Could you check a few things on this model? Use its own coordinates, in mm. Face numbers are marked on the shaded views. A direction names the side the tool comes from. Give positions to 0.01 mm unless a question says otherwise; leave off trailing zeros. Order: outer loops, then holes, each group sorted by start corner. A loop starts at its lowest first (then second) coordinate and runs counter-clockwise, first axis right, second up. Notation, with made-up numbers: M 38.25,84.5 L 53.25,84.5 A29 cw 53.25,110.5 Z; hole C 89.5,-18 d9. An arc over 180 degrees is marked long. Use a Markdown table: item, result. Add a question column.
Item 1: Suppose I cut it at A-A on z = -4. Write out the boundary of the cut face in (x, y), plus the area to 3 significant figures.
Item 2: Suppose I cut it at D-D on y = -12.5. Write out the boundary of the cut face in (x, z), plus the area to 3 significant figures.
Item 3: For the marked faces 1, 2 and 3, which set-ups out of +Z, -Z, +X, -X, +Y, -Y let a thin tool reach every point of the face, with its end or its side?
Item 4: Suppose I cut it at C-C on x = -9.5. Write out the boundary of the cut face in (y, z).
Item 5: If I drill on L1, parallel to Y at x = -12.9, z = -4; L2, parallel to Y at x = -1.25, z = 3; L3, parallel to X at y = -18.5, z = 0, over which ranges is the centre line in solid material (lowest first)? Write a range as from..to.
Item 6: Suppose I cut it at B-B on z = -7. Write out the boundary of the cut face in (x, y).
Item 7: I'm going to push flat-ended pins straight in: pin 1 Ø3 at (x, y) = (-6.31, 1.14) entering from -Z; pin 2 Ø2 at (x, y) = (-13.5, -30) entering from +Z; pin 3 Ø2 at (x, z) = (-9, 2) entering from -Y. Where does each tip first touch, or does it pass through?
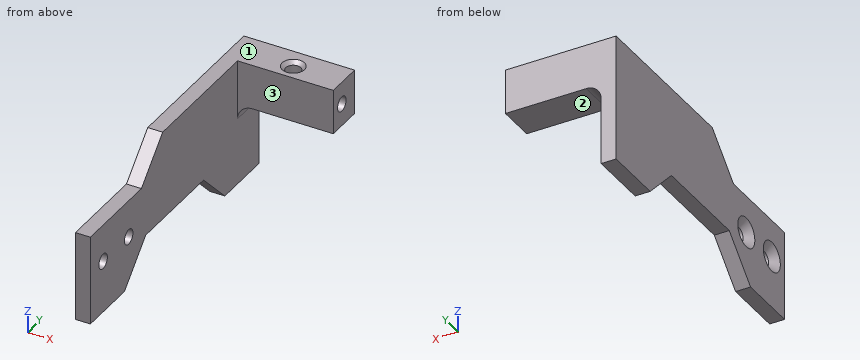
Autodesk Inventor part; units mm, degrees
ref_plane "YZ Plane" through (0, 0, 0) normal (1, 0, 0) x (0, 1, 0)
ref_plane "XZ Plane" through (0, 0, 0) normal (0, 1, 0) x (-1, 0, 0)
ref_plane "XY Plane" through (0, 0, 0) normal (0, 0, 1) x (1, 0, 0)
sketch "Sketch1" plane through (0, 0, 0) normal (0, 0, 1) x (1, 0, 0)
  line L0 (-12.5097, 3.9382) -> (-0.5097, 3.9382)
  line L1 (-0.5097, 3.9382) -> (-0.5097, -1.0618)
  line L2 (-0.5097, -1.0618) -> (-12.5097, -1.0618)
  line L3 (-12.5097, -1.0618) -> (-12.5097, 3.9382)
  point P0 (0, 0)
  dimension "d0" = 12
  dimension "d1" = 5
extrude "Extrusion1" add sketch "Sketch1" along normal blind 6
sketch "Sketch2" plane through (0, 0, 6) normal (0, 0, 1) x (1, 0, 0)
  line L0 (-0.5097, -1.0618) -> (-0.5097, 3.9382)
  line L1 (-0.5097, 3.9382) -> (-12.5097, 3.9382)
  point P0 (0, 0)
  point P1 (-6.3097, 1.1382)
  dimension "d4" = 5.8
  dimension "d5" = 2.8
hole "Hole1" at (-6.3097, 1.1382, 6) direction (0, 0, -1) diameter 2 depth 5 tip angle 118 countersink diameter 3 countersink angle 90
sketch "Sketch3" plane through (-0.5097, -1.0618, 0) normal (1, 0, 0) x (0, 0, -1)
  line L0 (0, 5) -> (-6, 5)
  line L1 (-6, 0) -> (-6, 5)
  point P0 (0, 1.0618)
  point P1 (-3, 2)
  dimension "d13" = 3
  dimension "d14" = 3
hole "Hole2" at (-0.5097, 0.9382, 3) direction (-1, 0, 0) diameter 2 depth 3 tip angle 118
sketch "Sketch4" plane through (-12.5097, -1.0618, 0) normal (-1, 0, 0) x (0, 0, 1)
  line L0 (6, 0) -> (6, 5)
  line L1 (6, 5) -> (-11, 5)
  line L2 (-11, 5) -> (-11, -34.6)
  line L3 (-11, -34.6) -> (6, -34.6)
  line L4 (6, -34.6) -> (6, 5)
  point P0 (0, 1.0618)
  dimension "d22" = 17
  dimension "d23" = 39.6
extrude "Extrusion2" add sketch "Sketch4" along normal blind 2
sketch "Sketch5" plane through (-14.5097, -1.0618, 0) normal (-1, 0, 0) x (0, 0, 1)
  line L0 (-11, -34.6) -> (6, -34.6)
  line L1 (6, -34.6) -> (6, 5)
  point P0 (0, 1.0618)
  point P1 (-4, -25.6)
  point P2 (-4, -31.6)
  dimension "d26" = 3
  dimension "d27" = 9
  dimension "d28" = 10
  dimension "d29" = 10
hole "Hole3" at (-14.5097, -26.6618, -4) at (-14.5097, -32.6618, -4) direction (1, 0, 0) diameter 2 depth 3 tip angle 118 countersink diameter 4 countersink angle 90
sketch "Sketch6" plane through (-0.5097, -1.0618, 0) normal (1, 0, 0) x (0, 0, -1)
  line L0 (-6, 5) -> (11, 5)
  line L1 (0, 5) -> (0, 0)
  line L2 (-6, 5) -> (0, 5)
  line L3 (0, 5) -> (0, 0)
  line L4 (0, 0) -> (-6, 0)
  line L5 (-6, 0) -> (-6, 5)
  circle A0 centre (-3, 2) radius 1
  circle A1 centre (-3, 2) radius 1
  point P0 (0, 1.0618)
  dimension "d37" = 2
extrude "Extrusion3" add sketch "Sketch6" along normal blind 0.8
sketch "Sketch7" plane through (-14.5097, -35.6618, 6) normal (-1, 0, 0) x (0, 0, 1)
  line L0 (-17, 39.6) -> (-17, 0)
  line L1 (-17, 31.6) -> (-12, 31.6)
  line L2 (-12, 31.6) -> (-12, 8)
  line L3 (-12, 8) -> (-17, 8)
  line L4 (-17, 8) -> (-17, 31.6)
  line L5 (0, 39.6) -> (-17, 39.6)
  line L6 (-17, 0) -> (0, 0)
  point P0 (-6, 35.6618)
  point P1 (-10, 0)
  point P2 (-17, 8)
  dimension "d40" = 5
  dimension "d41" = 8
  dimension "d42" = 8
extrude "Extrusion4" cut sketch "Sketch7" against normal blind 2
chamfer "Chamfer1" distance 5 angle 45 2 edges at (-13.5097, -4.0618, -6) (-13.5097, -27.6618, -6)
fillet "Fillet1" radius 2 1 edges at (-12.5097, 1.4382, 0)
sketch "Sketch8" plane through (-14.5097, -35.6618, 6) normal (-1, 0, 0) x (0, 0, 1)
  line L0 (0, 0) -> (0, 39.6)
  line L1 (-17, 0) -> (0, 0)
  line L2 (0, 12) -> (-5, 12)
  line L3 (-5, 12) -> (-5, 0)
  line L4 (-5, 0) -> (0, 0)
  line L5 (0, 0) -> (0, 12)
  point P0 (-6, 35.6618)
  point P1 (-10, 0)
  dimension "d49" = 5
  dimension "d50" = 12
extrude "Extrusion5" cut sketch "Sketch8" against normal blind 10
chamfer "Chamfer2" distance 5 angle 45 1 edges at (-13.5097, -23.6618, 6)
properties part number "servo-mount"
Findings below:
| question | item | result |
|---|---|---|
| 1 | outline | M -14.51,-35.66 L -12.51,-35.66 L -12.51,-33.66 L -13.51,-33.66 L -14.51,-34.66 Z; M -14.51,-30.66 L -13.51,-31.66 L -12.51,-31.66 L -12.51,-27.66 L -13.51,-27.66 L -14.51,-28.66 Z; M -14.51,-24.66 L -13.51,-25.66 L -12.51,-25.66 L -12.51,3.94 L -14.51,3.94 Z |
| 1 | area | 69.2 mm^2 |
| 2 | outline | M -14.51,-6 L -12.51,-6 L -12.51,6 L -14.51,6 Z |
| 2 | area | 24.0 mm^2 |
| 3 | face 1 | +Z, +X, -X, +Y, -Y |
| 3 | face 2 | -Z, +X, +Y, -Y |
| 3 | face 3 | +Z, -Z, +X, -Y |
| 4 | outline | M -1.06,0 L 3.94,0 L 3.94,6 L -1.06,6 Z |
| 5 | L1 | y = -35.66..-33.66, -31.66..-27.66, -25.66..3.94 |
| 5 | L2 | y = -1.06..-0.06, 1.94..3.94 |
| 5 | L3 | x = -14.51..-12.51 |
| 6 | outline | M -14.51,-35.66 L -12.51,-35.66 L -12.51,-23.66 L -14.51,-23.66 Z; M -14.51,-8.06 L -12.51,-8.06 L -12.51,3.94 L -14.51,3.94 Z |
| 7 | pin 1 | stops at z = 0 |
| 7 | pin 2 | stops at z = 1 |
| 7 | pin 3 | stops at y = -1.06 |
